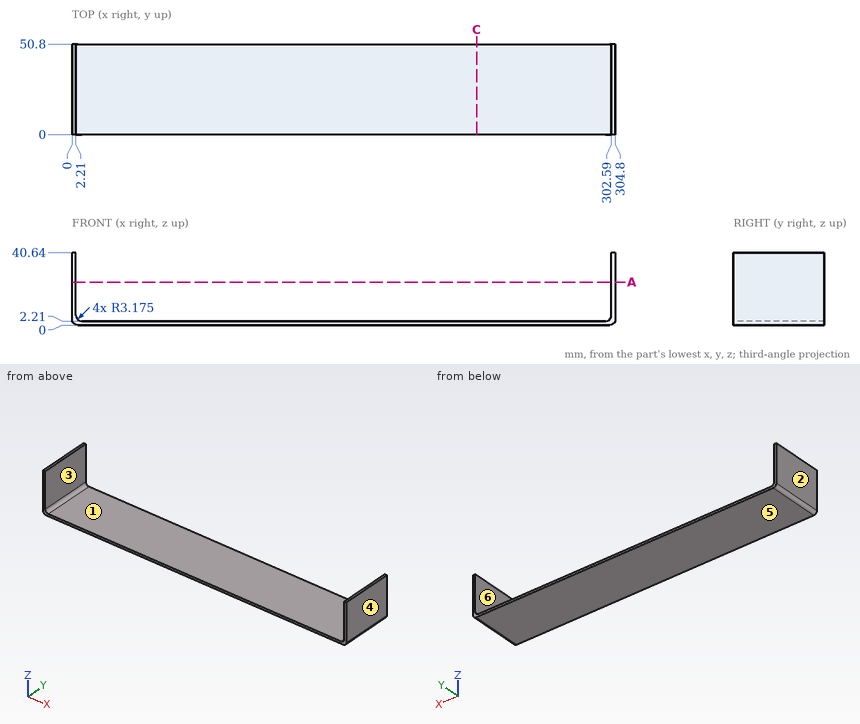
Geometry: see drawing. Coordinates: mm, zero at the bounding-box minimum. A direction names the side the tool comes from. Give positions to 0.01 mm unless a question says otherwise; leave off trailing zeros. Loops run counter-clockwise (first coordinate to the right, second up) from the corner with the lowest first, then second, coordinate; pieces in that order, holes last. Notation, with made-up numbers: M -30.75,3.25 L 23.25,3.25 A15 cw 23.25,13.25 Z; hole C 56.25,58.25 d7. An arc over 180 degrees is marked long. Answer as CSV lines item,"result". Start each with the question number.
1. Line query: L1, parallel to X at y = 33, z = 7.5; L2, parallel to Z at x = 133, y = 36; L3, parallel to X at y = 22, z = 4. Output: solid intervals per line, ascending.
2. Section A-A on z = 24. Return loops of the section in (x, y).
3. Pin query (flat end, axial travel): P1, Ø15, axis at x = 124.5, y = 19.5, coming from the +Z side. Return the tip coordinate at first contact, or that it passes through.
4. Section C-C on x = 227. Return loops of the section in (y, z), plus the area to 3 significant figures.
5. Reachability of the marked faces 5 and 6 from +Z, -Z, +X, -X, +Y, -Y: full face, straight path, thin tool, end or side. Return the list, or none.
6. Pull-direction query (X, two-part tool) for the marked faces 1, 2, 3 and 4; classes: released by +X, released by -X, zero draft, split by the parting line, or undercut.
Computed values:
1,L1,"x = 0 to 2.21, 302.59 to 304.8"
1,L2,"z = 0 to 2.21"
1,L3,"x = 0 to 2.53, 302.27 to 304.8"
2,outline,"M 0,0 L 2.21,0 L 2.21,50.8 L 0,50.8 Z; M 302.59,0 L 304.8,0 L 304.8,50.8 L 302.59,50.8 Z"
3,P1,"stops at z = 2.21"
4,outline,"M 0,0 L 50.8,0 L 50.8,2.21 L 0,2.21 Z"
4,area,"112 mm²"
5,face 5,"-Z, +X, -X, +Y, -Y"
5,face 6,"+Z, +Y, -Y"
6,face 1,"undercut"
6,face 2,"released by -X"
6,face 3,"undercut"
6,face 4,"released by +X"
